```python
from build123d import *

# Parameters (mm, degrees)
SKETCH1_R           = 1.2
SKETCH1_R_2         = 5
SKETCH1_W           = 13
SKETCH1_H           = 11
SKETCH1_W_2         = 10
SKETCH1_H_2         = 16
BOSS_EXTRUDE2_DEPTH = 3
SKETCH2_W           = 197.5
SKETCH2_H           = 78
BOSS_EXTRUDE3_DEPTH = 18
SKETCH3_W           = 191.5
SKETCH3_H           = 72
CUT_EXTRUDE1_DEPTH  = 1
SKETCH4_W           = 177.5
SKETCH4_H           = 55
CUT_EXTRUDE2_DEPTH  = 1
SKETCH5_W           = 11
SKETCH5_H           = 20
CUT_EXTRUDE3_DEPTH  = 8
SKETCH6_R           = 1
SKETCH6_W           = 7
SKETCH6_H           = 16
SKETCH6_W_2         = 5
SKETCH6_H_2         = 10
CUT_EXTRUDE4_DEPTH  = 10


with BuildPart() as part:
    # Sketch1 → Boss-Extrude2 (new body)
    with BuildSketch(Plane.XY):
        Polygon((0, 0), (197.5, 0), (197.5, 78), (0, 78), (0, 39), (8, 39), (8, 19), (0, 19), align=None)
        with Locations((37.25, 7.5)):
            Circle(SKETCH1_R, mode=Mode.SUBTRACT)
        with Locations((161.25, 7.5)):
            Circle(SKETCH1_R, mode=Mode.SUBTRACT)
        with Locations((156.5, 71)):
            Circle(SKETCH1_R, mode=Mode.SUBTRACT)
        with Locations((42, 71)):
            Circle(SKETCH1_R, mode=Mode.SUBTRACT)
        with Locations((23, 58)):
            Circle(SKETCH1_R_2, mode=Mode.SUBTRACT)
        with Locations((174.5, 57)):
            Circle(SKETCH1_R_2, mode=Mode.SUBTRACT)
        Polygon((47, 75), (47, 68), (40, 68), (40, 58), (47, 58), (47, 8), (144.5, 8), (144.5, 75), align=None, mode=Mode.SUBTRACT)
        with Locations((154, 62.5)):
            Rectangle(SKETCH1_W, SKETCH1_H, mode=Mode.SUBTRACT)
        with Locations((169.5, 14)):
            Rectangle(SKETCH1_W_2, SKETCH1_H_2, mode=Mode.SUBTRACT)
        with Locations((29, 14)):
            Rectangle(SKETCH1_W_2, SKETCH1_H_2, mode=Mode.SUBTRACT)
    extrude(amount=BOSS_EXTRUDE2_DEPTH)

    # Sketch2 → Boss-Extrude3 (add)
    with BuildSketch(Plane(origin=(0, 0, 0), x_dir=(-1, 0, 0), z_dir=(0, 0, -1))):
        with Locations((-98.75, 39)):
            Rectangle(SKETCH2_W, SKETCH2_H)
    extrude(amount=BOSS_EXTRUDE3_DEPTH)

    # Sketch3 → Cut-Extrude1 (cut)
    with BuildSketch(Plane(origin=(0, 0, -18), x_dir=(-1, 0, 0), z_dir=(0, 0, -1))):
        with Locations((-98.75, 39)):
            Rectangle(SKETCH3_W, SKETCH3_H)
    extrude(amount=-CUT_EXTRUDE1_DEPTH, mode=Mode.SUBTRACT)

    # Sketch4 → Cut-Extrude2 (cut)
    with BuildSketch(Plane(origin=(0, 0, -17), x_dir=(-1, 0, 0), z_dir=(0, 0, -1))):
        with Locations((-98.75, 42.5)):
            Rectangle(SKETCH4_W, SKETCH4_H)
    extrude(amount=-CUT_EXTRUDE2_DEPTH, mode=Mode.SUBTRACT)

    # Sketch5 → Cut-Extrude3 (cut)
    with BuildSketch(Plane.ZY):
        with Locations((-2.5, 29)):
            Rectangle(SKETCH5_W, SKETCH5_H)
    extrude(amount=-CUT_EXTRUDE3_DEPTH, mode=Mode.SUBTRACT)

    # Sketch6 → Cut-Extrude4 (cut)
    with BuildSketch(Plane(origin=(197.5, 0, 0), x_dir=(0, 0, -1), z_dir=(1, 0, 0))):
        with Locations((6, 66)):
            Circle(SKETCH6_R)
        with Locations((5.5, 15)):
            Rectangle(SKETCH6_W, SKETCH6_H)
        with Locations((6.5, 32)):
            Rectangle(SKETCH6_W_2, SKETCH6_H_2)
        with Locations((6.5, 48)):
            Rectangle(SKETCH6_W_2, SKETCH6_H_2)
    extrude(amount=-CUT_EXTRUDE4_DEPTH, mode=Mode.SUBTRACT)


solid = part.part
```
The model under review builds one solid part; all positions refer to its coordinate system, in mm. A direction names the side the tool comes from. Coordinates: 2 decimals unless noted, no trailing zeros. Write each loop counter-clockwise with the first axis right and the second up, starting at its lowest first coordinate (ties: lowest second). Pieces come first, ordered by that corner, then holes.
1) Clearance check with flat-ended pins moving along their axes: pin 1 Ø2 at (x, y) = (146.5, 42) entering from -Z; pin 2 Ø6 at (x, y) = (23, 58) entering from +Z; pin 3 Ø0.6 at (y, z) = (65.5, -6) entering from +X. State where each tip first meets the part, or that it passes through.
2) We need section B-B on x = 73. State the section outline as (y, z) points, then the cut area to 3 significant figures.
3) We need section A-A on y = 46. State the section outline as (x, z) points.
4) We need section C-C on y = 25. State the section outline as (x, z) points.
5) We need section D-D on x = 176.5. State the section outline as (y, z) points, then the cut area to 3 significant figures.
6) To check wall thickness, follow probe 1 along Y at (x, z) = (156.5, 0.9); probe 2 along X at (y, z) = (71, 0.7); probe 3 along Y at (x, z) = (42, 1.45). State the ranges of each line that lie inside material, in increasing order.
7) Machinability: for faces 4 (the face through (99, 77, -18)), 5 (the face through (100, 43, -16)), 6 (the face through (97, 5, 3)), 7 (the face through (22.349, 62.957, 1.479)), 8 (the face through (193, 37, -6)), which of the approach directions +Z, -Z, +X, -X, +Y, -Y give a long, thin tool a straight path to every point of the face, cutting with its end or side? Answer none if there is none.
8) The part is to be moulded in two halves that separate along Z. For faces 1 (the face through (0, 38, -10)), 2 (the face through (193, 53, -6)), 3 (the face through (23, 58, 0)), say which applies: pulls with the +Z half, pulls with the -Z half, needs draft (parallel to the pull), parting line crosses it, or undercut.
Answer list:
1. pin 1: stops at z = -16
1. pin 2: stops at z = 0
1. pin 3: stops at x = 187.5
2. outline: (0, -18) - (3, -18) - (3, -17) - (15, -17) - (15, -16) - (70, -16) - (70, -17) - (75, -17) - (75, -18) - (78, -18) - (78, 3) - (75, 3) - (75, 0) - (8, 0) - (8, 3) - (0, 3) - close
2. area: 1,310 mm2
3. outline: (0, -18) - (3, -18) - (3, -17) - (10, -17) - (10, -16) - (187.5, -16) - (187.5, -17) - (194.5, -17) - (194.5, -18) - (197.5, -18) - (197.5, -9) - (187.5, -9) - (187.5, -4) - (197.5, -4) - (197.5, 3) - (144.5, 3) - (144.5, 0) - (47, 0) - (47, 3) - (0, 3) - close
4. outline: (0, -18) - (3, -18) - (3, -17) - (10, -17) - (10, -16) - (187.5, -16) - (187.5, -17) - (194.5, -17) - (194.5, -18) - (197.5, -18) - (197.5, 3) - (144.5, 3) - (144.5, 0) - (47, 0) - (47, 3) - (8, 3) - (8, -8) - (0, -8) - close
5. outline: (0, -18) - (3, -18) - (3, -17) - (15, -17) - (15, -16) - (70, -16) - (70, -17) - (75, -17) - (75, -18) - (78, -18) - (78, 3) - (61.58, 3) - (61.58, 0) - (52.42, 0) - (52.42, 3) - (0, 3) - close
5. area: 1,480 mm2
6. probe 1: y = 0 to 57, 68 to 69.8, 72.2 to 78
6. probe 2: x = 0 to 40.8, 43.2 to 47, 144.5 to 155.3, 157.7 to 197.5
6. probe 3: y = 0 to 58, 68 to 69.8, 72.2 to 78
7. face 4: -Z, +X, -X, +Y, -Y
7. face 5: -Z
7. face 6: +Z, +X, -X, +Y, -Y
7. face 7: +Z
7. face 8: +X
8. face 1: needs draft
8. face 2: undercut
8. face 3: pulls with the +Z half
